Source: three-view drawing plus pictorial views. Frame: mm from the lowest corner of the part. A direction names the side the tool comes from. Give positions to 0.01 mm unless a question says otherwise; leave off trailing zeros. Loops run counter-clockwise (first coordinate to the right, second up) from the corner with the lowest first, then second, coordinate; pieces in that order, holes last. Notation, with made-up numbers: (-13.75, 10.5) - (42.25, 10.5) arc R29 cw to (42.25, 30.5) - close; hole circle Ø2 at (59.5, 62). An arc over 180 degrees is marked (long way). Answer in a Markdown table with one row per item.
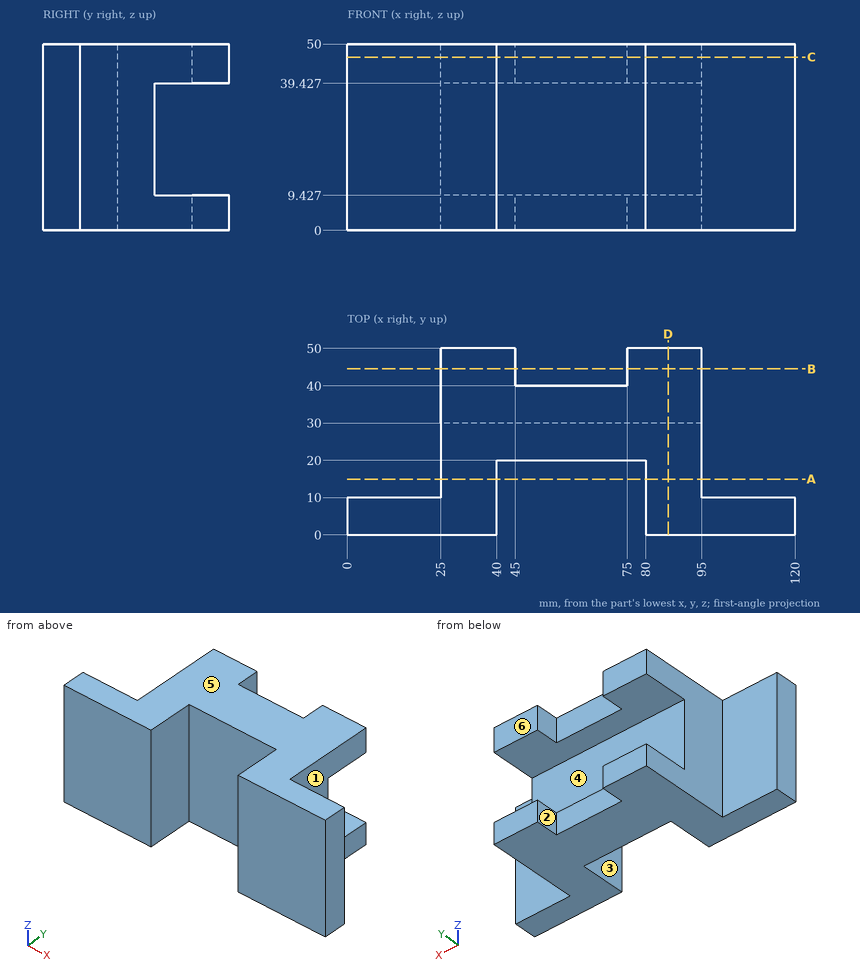
Q1. Cut plane A-A (y = 15). Output: boundary loops of the cut face in (x, z), and give its area (3 significant figures).
Check values:
| item | result |
|---|---|
| outline | (25, 0) - (40, 0) - (40, 50) - (25, 50) - close; (80, 0) - (95, 0) - (95, 50) - (80, 50) - close |
| area | 1,500 mm² |
Q2. Material intervals for line 1 along X through (y, z) = (3.5, 35.5); line 2 along Z through (x, y) = (40, 41.5); line 3 along X through (y, z) = (18.5, 46), sorted ascending.
Check values:
| item | result |
|---|---|
| line 1 | 0 to 40, 80 to 120 |
| line 2 | 0 to 9.43, 39.43 to 50 |
| line 3 | 25 to 40, 80 to 95 |
Q3. Cut plane D-D (x = 86). Output: boundary loops of the cut face in (y, z).
Check values:
| item | result |
|---|---|
| outline | (0, 0) - (50, 0) - (50, 9.43) - (30, 9.43) - (30, 39.43) - (50, 39.43) - (50, 50) - (0, 50) - close |
Q4. Cut plane B-B (y = 44.5). Output: boundary loops of the cut face in (x, z).
Check values:
| item | result |
|---|---|
| outline | (25, 0) - (45, 0) - (45, 9.43) - (25, 9.43) - close; (25, 39.43) - (45, 39.43) - (45, 50) - (25, 50) - close; (75, 0) - (95, 0) - (95, 9.43) - (75, 9.43) - close; (75, 39.43) - (95, 39.43) - (95, 50) - (75, 50) - close |
Q5. First-contact query: pin 1 (20 mm diameter, centred on x = 104.5, z = 23, fed in from +Y); pin 2 (8.5 mm diameter, centred on x = 54.5, z = 43, fed in from +Y); pin 3 (3 mm diameter, centred on y = 46, z = 3.5, fed in from +X). Flat tips, straight axial feed; report the tip coordinate or a pass-through.
Check values:
| item | result |
|---|---|
| pin 1 | y = 30 |
| pin 2 | y = 40 |
| pin 3 | x = 95 |
Q6. Reachability of the marked faces 1, 2 and 3 from +Z, -Z, +X, -X, +Y, -Y: full face, straight path, thin tool, end or side. Return the list, or none.
Check values:
| item | result |
|---|---|
| face 1 | +Z, -Z, +X, +Y |
| face 2 | +Z, -Z, +Y |
| face 3 | +Z, -Z, -Y |
Q7. Draft query along Z for the marked faces 4, 5 and 6. Return one class per face: pulls with the +Z half, pulls with the -Z half, needs draft (parallel to the pull), parting line crosses it, or undercut.
Check values:
| item | result |
|---|---|
| face 4 | undercut |
| face 5 | pulls with the +Z half |
| face 6 | needs draft |
Q8. Cut plane C-C (z = 46.5). Output: boundary loops of the cut face in (x, y), and give its area (3 significant figures).
Check values:
| item | result |
|---|---|
| outline | (0, 0) - (40, 0) - (40, 20) - (80, 20) - (80, 0) - (120, 0) - (120, 10) - (95, 10) - (95, 50) - (75, 50) - (75, 40) - (45, 40) - (45, 50) - (25, 50) - (25, 10) - (0, 10) - close |
| area | 2,900 mm² |
